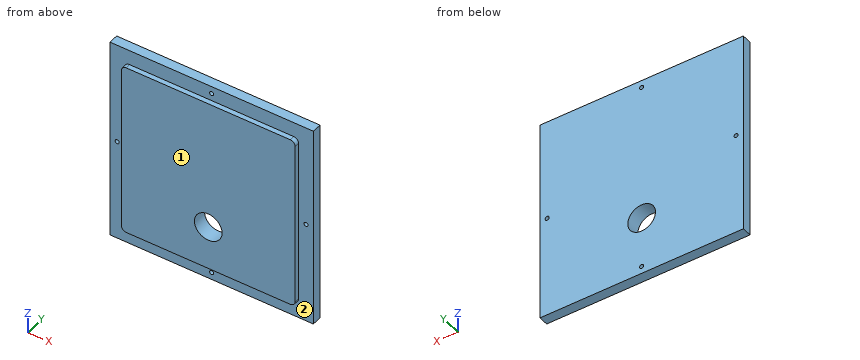
from build123d import *

# Parameters (mm, degrees)
SKETCH2_W           = 210
SKETCH2_H           = 210
BOSS_EXTRUDE1_DEPTH = 10
SKETCH3_W           = 179.6
SKETCH3_H           = 179.6
BOSS_EXTRUDE2_DEPTH = 5
BOSS_EXTRUDE2_TAPER = 2
SKETCH4_R           = 14.3
CUT_EXTRUDE1_DEPTH  = 15
SKETCH6_R           = 2.1
CUT_EXTRUDE2_DEPTH  = 10
FILLET1_R           = 5


with BuildPart() as part:
    # Sketch2 → Boss-Extrude1 (new body)
    with BuildSketch(Plane(origin=(0, 0, 0), x_dir=(1, 0, 0), z_dir=(0, 1, 0))):
        Rectangle(SKETCH2_W, SKETCH2_H)
    extrude(amount=BOSS_EXTRUDE1_DEPTH)

    # Sketch3 → Boss-Extrude2 (add)
    with BuildSketch(Plane.XZ):
        Rectangle(SKETCH3_W, SKETCH3_H)
    extrude(amount=BOSS_EXTRUDE2_DEPTH, taper=BOSS_EXTRUDE2_TAPER)

    # Sketch4 → Cut-Extrude1 (cut)
    with BuildSketch(Plane(origin=(0, 10, 0), x_dir=(1, 0, 0), z_dir=(0, 1, 0))):
        with Locations((0, 44.625396153)):
            Circle(SKETCH4_R)
    extrude(amount=-CUT_EXTRUDE1_DEPTH, mode=Mode.SUBTRACT)

    # Sketch6 → Cut-Extrude2 (cut)
    with BuildSketch(Plane(origin=(0, 10, 0), x_dir=(1, 0, 0), z_dir=(0, 1, 0))):
        with Locations((0, 97.5)):
            Circle(SKETCH6_R)
        with Locations((-97.5, 0)):
            Circle(SKETCH6_R)
        with Locations((0, -97.5)):
            Circle(SKETCH6_R)
        with Locations((97.5, 0)):
            Circle(SKETCH6_R)
        with Locations((0, 97.5)):
            Circle(SKETCH6_R)
        with Locations((0, 97.5)):
            Circle(SKETCH6_R)
        with Locations((0, 97.5)):
            Circle(SKETCH6_R)
    extrude(amount=-CUT_EXTRUDE2_DEPTH, mode=Mode.SUBTRACT)

    # Fillet1
    fillet1_edges = [part.edges().sort_by_distance(p)[0] for p in [
        (89.712698076, -2.5, -89.712698076),
        (89.712698076, -2.5, 89.712698076),
        (-89.712698076, -2.5, 89.712698076),
        (-89.712698076, -2.5, -89.712698076),
    ]]
    fillet(fillet1_edges, radius=FILLET1_R)


solid = part.part
Geometry check sheet. Reference: the model listing, model coordinates, mm. Face numbers are marked on the shaded views. A direction names the side the tool comes from. Coordinates: 2 decimals unless noted, no trailing zeros. Loops run counter-clockwise (first coordinate to the right, second up) from the corner with the lowest first, then second, coordinate; pieces in that order, holes last. Notation, with made-up numbers: (-35.5, -16.75) - (15.5, -16.75) arc R8 cw to (15.5, -2.75) - close; hole circle Ø10 at (20.25, -37.75). An arc over 180 degrees is marked (long way). Use one line per item in the form item = value. Start each with the question number.
Item 1: Gauge pin test, flat end, axial feed: pin 1 (4 mm diameter, centred on x = 97.5, z = 0, fed in from +Y). Record the tip position at first contact, or that the pin passes through.
Item 2: Section check A-A, the plane y = 6.75. Enter the section's corners in (x, z).
Item 3: Thickness scan on probe 1 along X at (y, z) = (4.25, 0); probe 2 along Z at (x, y) = (-97.5, 5); probe 3 along Z at (x, y) = (0, 7.5). Record the ranges inside material, lowest first.
Item 4: Tool access check on the marked faces 1 and 2. Record the directions out of +Z, -Z, +X, -X, +Y, -Y that give a thin tool (end or side, any length) a straight path to the whole face; none if there is none.
Computed:
q1.pin_1 = through
q2.outline = (-105, -105) - (105, -105) - (105, 105) - (-105, 105) - close; hole circle Ø4.2 at (-97.5, 0); hole circle Ø28.6 at (0, -44.63); hole circle Ø4.2 at (0, -97.5); hole circle Ø4.2 at (0, 97.5); hole circle Ø4.2 at (97.5, 0)
q3.probe_1 = -105 to -99.6, -95.4 to 95.4, 99.6 to 105
q3.probe_2 = -105 to -2.1, 2.1 to 105
q3.probe_3 = -105 to -99.6, -95.4 to -58.93, -30.33 to 95.4, 99.6 to 105
q4.face_1 = +Z, -Z, +X, -X, -Y
q4.face_2 = -Y
